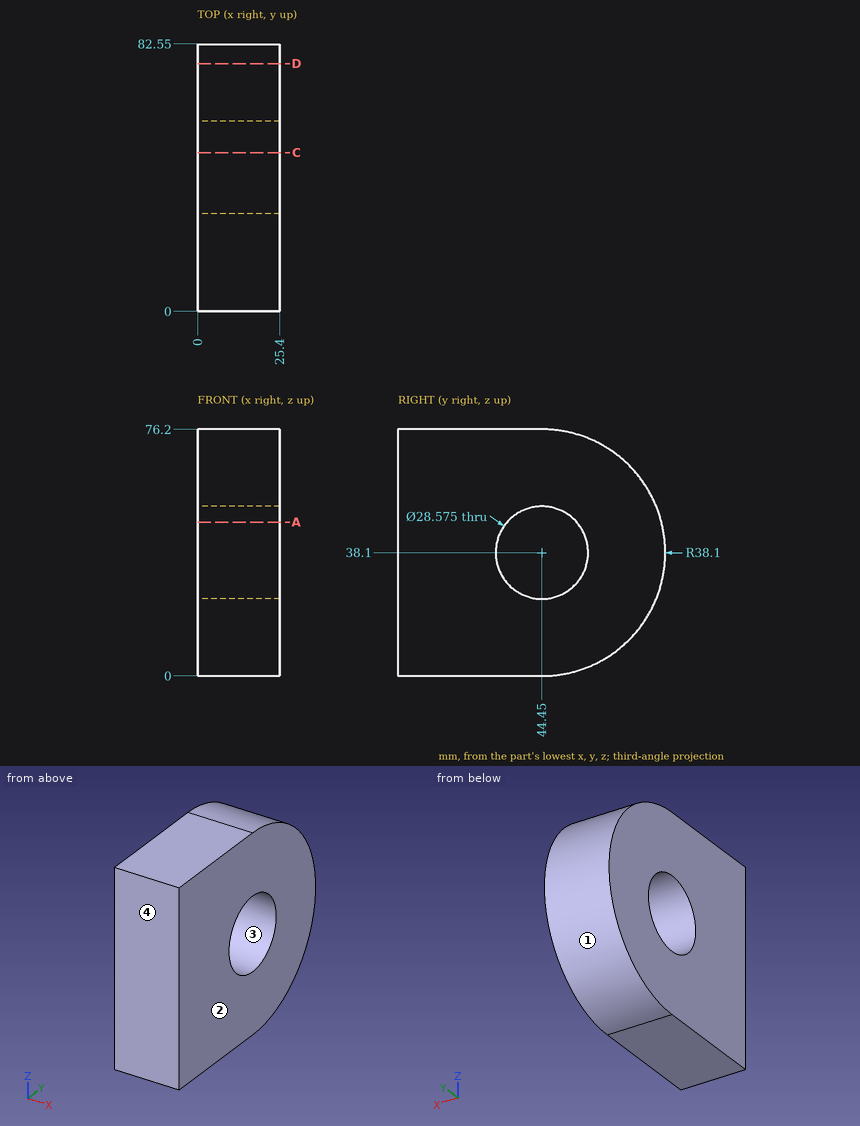
Drawing for the job (mm, zero at the part's lowest x, y, z). Give positions to 0.01 mm unless a question says otherwise; leave off trailing zeros. Order: outer loops, then holes, each group sorted by start corner. A loop starts at its lowest first (then second) coordinate and runs counter-clockwise, first axis right, second up. Notation, with made-up numbers: M 38.25,80 L 62.25,80 A22 cw 62.25,113 Z; hole C -33,-0.75 d7. An arc over 180 degrees is marked long. Put each result on its own line as item: value. Start each with the question number.
(1) Flat gauge pins, fed straight in: pin 1 Ø2 at (y, z) = (23.5, 54.5) entering from -X; pin 2 Ø23 at (y, z) = (44.45, 38.1) entering from -X; pin 3 Ø4 at (x, y) = (8, 50.5) entering from +Z; pin 4 Ø2 at (x, y) = (21, 61.5) entering from -Z. Where does each tip first touch, or does it go through?
(2) Saw through at A-A, the plane z = 47.5. Write the cut outline in (x, y).
(3) Drill centre lines: line 1 along Y through (x, z) = (11.75, 38.1); line 2 along Z through (x, y) = (13, 47); line 3 along Y through (x, z) = (12, 42). Where is each one in solid material? Low to high.
(4) Saw through at C-C, the plane y = 49. Write the cut outline in (x, z).
(5) Saw through at D-D, the plane y = 76.5. Write the cut outline in (x, z).
(6) Mould opens along Y. For the marked faces 1, 2, 3 and 4 say: +Y half, -Y half, draft (parallel to the pull), parting line (faces both ways), or undercut.
Check result:
1. pin 1: stops at x = 0
1. pin 2: passes through
1. pin 3: stops at z = 75.98
1. pin 4: stops at z = 3.55
2. outline: M 0,0 L 25.4,0 L 25.4,33.69 L 0,33.69 Z; M 0,55.21 L 25.4,55.21 L 25.4,81.37 L 0,81.37 Z
3. line 1: y = 0 to 30.16, 58.74 to 82.55
3. line 2: z = 0.09 to 24.04, 52.16 to 76.11
3. line 3: y = 0 to 30.71, 58.19 to 82.35
4. outline: M 0,0.27 L 25.4,0.27 L 25.4,24.56 L 0,24.56 Z; M 0,51.64 L 25.4,51.64 L 25.4,75.93 L 0,75.93 Z
5. outline: M 0,17.5 L 25.4,17.5 L 25.4,58.7 L 0,58.7 Z
6. face 1: +Y half
6. face 2: draft
6. face 3: undercut
6. face 4: -Y half
